Geometry: final body of the model. Coordinates: model frame, mm. A direction names the side the tool comes from. Give positions to 0.01 mm unless a question says otherwise; leave off trailing zeros. Loops run counter-clockwise (first coordinate to the right, second up) from the corner with the lowest first, then second, coordinate; pieces in that order, holes last.
1. Draft query along X for faces 4 (the face through (2, 0, -4)), 5 (the face through (-3.744, -6.219, 0.125)), 6 (the face through (-6.55, -9.39, 6.01)). Return one class per face: +X half, -X half, draft (parallel to the pull), parting line (faces both ways), or undercut.
2. Material intervals for line 1 along Y through (x, z) = (0, 3.5) (3 decimals); line 2 along Y through (x, z) = (0, -4.75); line 3 along Y through (x, z) = (-7.75, 2.75), sorted ascending.
3. Access query for faces 1 (the face through (0, -22.225, 0)), 2 (the face through (0.86, 1.565, -3.874)), 3 (the face through (-0.86, -20.615, -3.874)). Directions: +Z, -Z, +X, -X, +Y, -Y. A direction counts if a zero-diameter tool reaches every point of the face in a straight line with its end or side. Return the directions, or none.
4. Section C-C, the plane y = -3.25. Output: boundary loops of the cut face in (x, z), then the cut area to 3 significant figures.
5. Section B-B, the plane z = 0. Output: boundary loops of the cut face in (x, y) (3 decimals).
6. Section A-A, the plane x = 0. Output: boundary loops of the cut face in (y, z) (3 decimals), then the cut area to 3 significant figures.
7. Section D-D, the plane y = -11.25. Output: boundary loops of the cut face in (x, z).
8. First-contact query: P1, Ø9, axis at x = 0, y = -9.652, coming from the -Z side; P2, Ø2, axis at y = -10, z = -4, coming from the +X side; P3, Ø2, axis at y = -8.5, z = -2, coming from the -X side; P4, Ø2, axis at x = 3.5, y = -19, coming from the +Z side. Flat tips, straight axial feed; report the tip coordinate or a pass-through.
from build123d import *

# Parameters (mm, degrees)
F0_R     = 8.89
F1_DEPTH = 19.05
F2_R     = 3.96875
F3_DEPTH = 3.175
F4_R     = 3.96875
F5_DEPTH = 3.175
F7_R     = 5.08
F8_DEPTH = 25.4


with BuildPart() as f1:
    # F0 (on Front) → F1 (new body)
    with BuildSketch(Plane.XZ):
        Circle(F0_R)
    extrude(amount=F1_DEPTH)

    # F2 (on face) → F3 (join)
    with BuildSketch(Plane.XZ.offset(19.05)):
        Circle(F2_R)
    extrude(amount=F3_DEPTH)

    # F4 (on face) → F5 (join)
    with BuildSketch(Plane(origin=(0, 0, 0), x_dir=(-1, 0, 0), z_dir=(0, 1, 0))):
        Circle(F4_R)
    extrude(amount=F5_DEPTH)

    # F7 (on offset) → F8 (cut)
    with BuildSketch(Plane.XY.offset(10.16)):
        with Locations((0, -9.652)):
            Circle(F7_R)
    extrude(amount=-F8_DEPTH, mode=Mode.SUBTRACT)


solid = f1.part
Answers below:
1. face 4: draft
1. face 5: undercut
1. face 6: parting line
2. line 1: y = -22.225 to -14.732, -4.572 to 3.175
2. line 2: y = -19.05 to -14.73, -4.57 to 0
2. line 3: y = -19.05 to 0
3. face 1: +Z, -Z, +X, -X, -Y
3. face 2: +Y
3. face 3: -Y
4. outline: circle Ø17.78 at (0, 0)
4. area: 248 mm2
5. outline: (-8.89, -19.05) - (-3.969, -19.05) - (-3.969, -22.225) - (3.969, -22.225) - (3.969, -19.05) - (8.89, -19.05) - (8.89, 0) - (3.969, 0) - (3.969, 3.175) - (-3.969, 3.175) - (-3.969, 0) - (-8.89, 0) - close; hole circle Ø10.16 at (0, -9.652)
6. outline: (-22.225, -3.969) - (-19.05, -3.969) - (-19.05, -8.89) - (-14.732, -8.89) - (-14.732, 8.89) - (-19.05, 8.89) - (-19.05, 3.969) - (-22.225, 3.969) - close; (-4.572, -8.89) - (0, -8.89) - (0, -3.969) - (3.175, -3.969) - (3.175, 3.969) - (0, 3.969) - (0, 8.89) - (-4.572, 8.89) - close
6. area: 208 mm2
7. outline: (-4.82, -7.47) - (-4.82, 7.47) arc R8.89 ccw to start; (4.82, -7.47) arc R8.89 ccw to (4.82, 7.47) - close
8. P1: passes through
8. P2: stops at x = 8.37
8. P3: stops at x = -8.83
8. P4: stops at z = 8.53
